from build123d import *

# Parameters (mm, degrees)
F0_R     = 70
F0_R_2   = 5
F1_DEPTH = 7
F2_R     = 50
F2_R_2   = 44
F3_DEPTH = 18
F4_R     = 44
F5_DEPTH = 2
F6_R     = 3


with BuildPart() as f1:
    # F0 (on Top) → F1 (new body)
    with BuildSketch(Plane.XY):
        Circle(F0_R)
        with Locations((0, -61)):
            Circle(F0_R_2, mode=Mode.SUBTRACT)
        with Locations((-61, 0)):
            Circle(F0_R_2, mode=Mode.SUBTRACT)
        with Locations((61, 0)):
            Circle(F0_R_2, mode=Mode.SUBTRACT)
        with Locations((0, 61)):
            Circle(F0_R_2, mode=Mode.SUBTRACT)
    extrude(amount=F1_DEPTH)

    # F2 (on face) → F3 (join)
    with BuildSketch(Plane.XY.offset(7)):
        Circle(F2_R)
        Circle(F2_R_2, mode=Mode.SUBTRACT)
    extrude(amount=F3_DEPTH)

    # F4 (on face) → F5 (cut)
    with BuildSketch(Plane.XY.offset(7)):
        Circle(F4_R)
    extrude(amount=-F5_DEPTH, mode=Mode.SUBTRACT)

    # F6
    f6_edges = [f1.edges().sort_by_distance(p)[0] for p in [
        (-44, 0, 5),
    ]]
    fillet(f6_edges, radius=F6_R)


solid = f1.part
Read the model definition and answer for the solid it produces. Units are mm, in the model's axes. A direction names the side the tool comes from. Round coordinates to 2 decimals unless told otherwise and drop trailing zeros. Write each loop counter-clockwise with the first axis right and the second up, starting at its lowest first coordinate (ties: lowest second). Pieces come first, ordered by that corner, then holes. Notation, with made-up numbers: (-17, 0.5) - (17, 0.5) arc R18 ccw to (17, 7.5) - close; hole circle Ø9 at (-0.5, 2). An arc over 180 degrees is marked (long way). One line per question, with ' | ' between items. Start each with the question number.
1. For a pull along X with two mould halves and no side action, classify faces 3 (the face through (-55.55, -42.594, 3.451)), 4 (the face through (3, 65, 3)), 5 (the face through (-1, 1, 0)) as +X half, -X half, draft (parallel to the pull), parting line (faces both ways), or undercut.
2. For faces 1 (the face through (-9.538, -42.954, 16.381)), 2 (the face through (56, 0, 3)), determine the directions among +Z, -Z, +X, -X, +Y, -Y from which every point of the face is accessible in a straight line to the end or side of a thin tool.
3. Each of these flat-tipped pins is pushed along its axis until it touches: pin 1 (11.5 mm diameter, centred on x = -61, y = 0, fed in from +Z); pin 2 (5 mm diameter, centred on y = 19, z = 7.5, fed in from +X); pin 3 (2 mm diameter, centred on y = -30, z = 5.5, fed in from -X). Where does it stop, or does it pass through?
4. Section C-C (x = -61) is taken. Determine the outline of the cut face in (y, z), and give its area (3 significant figures).
5. Section A-A (x = 0) is taken. Determine the outline of the cut face in (y, z).
6. Find the intervals of material crossed by probe 1 along Y at (x, z) = (0, 17.5); probe 2 along Y at (x, z) = (0, 5.25); probe 3 along Z at (x, y) = (-2.5, 54.5), in increasing order. Write a range as [from, to].
Filled in:
1) face 3: parting line | face 4: undercut | face 5: draft
2) face 1: +Z | face 2: +Z, -Z
3) pin 1: z = 7 | pin 2: x = 68.02 | pin 3: x = -63.71
4) outline: (-34.34, 0) - (-5, 0) - (-5, 7) - (-34.34, 7) - close; (5, 0) - (34.34, 0) - (34.34, 7) - (5, 7) - close | area: 411 mm²
5) outline: (-70, 0) - (-66, 0) - (-66, 7) - (-70, 7) - close; (-56, 0) - (56, 0) - (56, 7) - (50, 7) - (50, 25) - (44, 25) - (44, 8) arc R3 cw to (41, 5) - (-41, 5) arc R3 cw to (-44, 8) - (-44, 25) - (-50, 25) - (-50, 7) - (-56, 7) - close; (66, 0) - (70, 0) - (70, 7) - (66, 7) - close
6) probe 1: [-50, -44], [44, 50] | probe 2: [-70, -66], [-56, -42.2], [42.2, 56], [66, 70] | probe 3: [0, 7]
